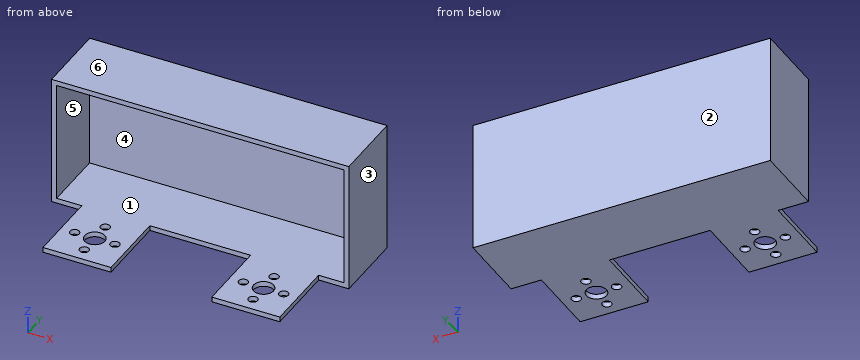
Autodesk Inventor part; units mm, degrees
ref_plane "YZ Plane" through (0, 0, 0) normal (1, 0, 0) x (0, 1, 0)
ref_plane "XZ Plane" through (0, 0, 0) normal (0, 1, 0) x (-1, 0, 0)
ref_plane "XY Plane" through (0, 0, 0) normal (0, 0, 1) x (1, 0, 0)
ref_plane "Work Plane7" through (-37.2167, 31.2213, -6.3329) normal (0, 1, 0) x (1, 0, 0)
sketch "Sketch1" plane through (-37.2167, 31.2213, -6.3329) normal (0, 1, 0) x (1, 0, 0)
  arc A0 (-58.7242, 8.25) -> (-74.6429, -6.8045) centre (-66, 0) ccw
  line L0 (-77, 0) -> (-77, -32.6485)
  arc A1 (-74.6429, -15.1955) -> (-58.7242, -30.25) centre (-66, -22) ccw
  line L1 (-66, -33) -> (-77, -33)
  line L2 (-77, -32.6485) -> (-77, -33)
  line L3 (-77, 0) -> (-77, 11)
  arc A2 (30, -7.5498) -> (14.7242, 8.25) centre (22, 0) ccw
  line L4 (22, 11) -> (-77, 11)
  line L5 (-66, -33) -> (33, -33)
  arc A3 (14.7242, -30.25) -> (30, -14.4502) centre (22, -22) ccw
  line L6 (33, -22) -> (33, -33)
  line L7 (33, -22) -> (33, 11)
  line L8 (22, 11) -> (33, 11)
  line L9 (-79, -32.6485) -> (-79, 0)
  line L10 (-79, 0) -> (-79, 13)
  line L11 (-79, 13) -> (22, 13)
  line L12 (22, 13) -> (35, 13)
  line L13 (35, 13) -> (35, -22)
  line L14 (35, -22) -> (35, -35)
  line L15 (35, -35) -> (-66, -35)
  line L16 (-66, -35) -> (-79, -35)
  line L17 (-79, -35) -> (-79, -32.6485)
  line L18 (-81, 15) -> (-81, 0)
  line L19 (-81, 0) -> (-81, -32.6485)
  line L20 (-81, -32.6485) -> (-81, -37)
  line L21 (-81, -37) -> (-66, -37)
  line L22 (-66, -37) -> (37, -37)
  line L23 (37, -37) -> (37, -22)
  line L24 (37, -22) -> (37, 15)
  line L25 (37, 15) -> (22, 15)
  line L26 (22, 15) -> (-81, 15)
  point P0 (37.2167, -6.3329)
  dimension "d0" = 2
  dimension "d1" = 4
extrude "Extrusion1" add sketch "Sketch1" against normal blind 25 contours L26 L25 L24 L23 L22 L21 L20 L19 L18
extrude "Extrusion2" add sketch "Sketch1" along normal blind 4 contours L4 A2 L7 A3 L5 A1 L0 A0 | A0 L3 L4 | L8 L7 A2 | A1 L1 L2 L0 | L6 L5 A3 | L9 L10 L11 L12 L13 L14 L15 L16 L17 | L26 L25 L24 L23 L22 L21 L20 L19 L18
sketch "Sketch3" plane through (-118.2167, 6.2213, 30.6671) normal (0, 0, 1) x (1, 0, 0)
  point P0 (118.2167, -6.2213)
sketch "Sketch4" plane through (-118.2167, 6.2213, 30.6671) normal (0, 0, 1) x (1, 0, 0)
  point P0 (118.2167, -6.2213)
ref_plane "Work Plane2" through (-37.2167, 6.2213, -6.3329) normal (0, -1, 0) x (1, 0, 0)
sketch "Sketch5" plane through (-37.2167, 6.2213, -6.3329) normal (0, -1, 0) x (1, 0, 0)
  line L0 (35, -13) -> (-79, -13)
  line L1 (35, -13) -> (35, -15)
  line L2 (-81, -15) -> (37, -15)
  line L3 (-79, 35) -> (-79, -13)
  line L4 (-79, -13) -> (-79, -15)
  line L5 (-79, -15) -> (35, -15)
  line L6 (35, -15) -> (25, -15)
  line L7 (25, -15) -> (25, -13)
  line L8 (25, -13) -> (-2, -13)
  line L9 (-2, -13) -> (-2, -15)
  line L10 (25, -15) -> (-2, -15)
  line L11 (-79, -15) -> (-69, -15)
  line L12 (-69, -15) -> (-69, -13)
  line L13 (-69, -13) -> (-42, -13)
  line L14 (-42, -13) -> (-42, -15)
  line L15 (-69, -15) -> (-42, -15)
  point P0 (37.2167, 6.3329)
  point P1 (-2, -15)
  point P2 (25, -15)
  point P3 (-42, -15)
  point P4 (-69, -15)
  dimension "d30" = 10
  dimension "d31" = 27
  dimension "d32" = 10
  dimension "d33" = 27
extrude "Extrusion3" add sketch "Sketch5" along normal blind 29.5 contours L7 L2 L9 L0 | L14 L2 L12 L0
ref_plane "Work Plane3" through (-0.2167, 35.2213, -21.3329) normal (0, 0, -1) x (-1, 0, 0)
sketch "Sketch6" plane through (-0.2167, 35.2213, -21.3329) normal (0, 0, -1) x (-1, 0, 0)
  line L0 (106, -58.5) -> (79, -58.5)
  line L1 (106, -58.5) -> (92.5, -58.5)
  line L2 (92.5, -58.5) -> (92.5, -53)
  circle A0 centre (92.5, -53) radius 1.85
  line L3 (92.5, -53) -> (92.5, -45)
  circle A1 centre (92.5, -45) radius 4
  line L4 (92.5, -45) -> (92.5, -37)
  circle A2 centre (92.5, -37) radius 1.85
  line L5 (92.5, -45) -> (84.5, -45)
  line L6 (93.7399, -45) -> (90.2601, -45)
  line L7 (84.5, -45) -> (100.5, -45)
  circle A3 centre (100.5, -45) radius 1.85
  circle A4 centre (84.5, -45) radius 1.85
  line L8 (79, -29) -> (39, -29)
  line L9 (79, -29) -> (59, -29)
  line L10 (59, -29) -> (59, -58.5)
  circle A5 centre (25.5, -53) radius 1.85
  circle A6 centre (25.5, -45) radius 4
  circle A7 centre (25.5, -37) radius 1.85
  circle A8 centre (17.5, -45) radius 1.85
  circle A9 centre (33.5, -45) radius 1.85
  point P0 (-0.2167, -35.2213)
  dimension "d36" = 5.5
  dimension "d37" = 3.7
  dimension "d38" = 8
  dimension "d39" = 8
  dimension "d40" = 8
  dimension "d41" = 3.7
  dimension "d42" = 8
  dimension "d43" = 16
  dimension "d44" = 3.7
  dimension "d45" = 3.7
  dimension "d46" = 20
extrude "Extrusion4" cut sketch "Sketch6" against normal blind 2.25
properties part number "39057 TETRIX 12V 3000mAH Battery Pack Assembly"
Read the model definition and answer for the solid it produces. Units are mm, in the model's axes. Face numbers are marked on the shaded views. A direction names the side the tool comes from. Coordinates: 2 decimals unless noted, no trailing zeros. Order: outer loops, then holes, each group sorted by start corner. A loop starts at its lowest first (then second) coordinate and runs counter-clockwise, first axis right, second up. Notation, with made-up numbers: (43.25, 82) - (61.25, 82) arc R16 ccw to (61.25, 95) - close; hole circle Ø2 at (65.5, 33). An arc over 180 degrees is marked (long way). Answer as a JSON object with one key per item and string values. Group by question number.
Item 1: Section C-C (x = -108) is taken. Give the vertices of the cut face in (y, z), plus the area to 3 significant figures.
Item 2: Flat-ended cylindrical pins translate along their axes: P1, Ø13, axis at x = -25.72, y = -9.78, coming from the -Z side; P2, Ø1.5, axis at x = -85, z = -16, coming from the -Y side; P3, Ø2, axis at x = -55, z = -20.5, coming from the -Y side; P4, Ø1, axis at y = -13, z = -20, coming from the -X side. Find the tip coordinate at first contact, or state that the pin passes through.
Item 3: Section A-A (y = 30) is taken. Give the vertices of the cut face in (x, z), plus the area to 3 significant figures.
Item 4: A tool of negligible diameter and unlimited length cuts with its end or side. For the marked faces 1 and 2, from which of +Z, -Z, +X, -X, +Y, -Y can it reach the whole face along a straight path? Write none if from no direction.
Item 5: Consider probe 1 along Z at (x, y) = (-82, 21); probe 2 along X at (y, z) = (22, 9.5); probe 3 along Y at (x, z) = (-59, 16.5). Determine where each line is inside the solid, lowest interval first. Write a range as from..to.
Item 6: Section D-D (z = 19) is taken. Give the vertices of the cut face in (x, y).
Item 7: The mould has two halves that part along X. Classify the marked faces 3, 4, 5 and 6: +X half, -X half, draft (parallel to the pull), parting line (faces both ways), or undercut.
Item 8: Section B-B (y = 1.5) is taken. Give the vertices of the cut face in (x, z).
Results are:
{
 "1": {"outline": "(6.22, -21.33) - (35.22, -21.33) - (35.22, 30.67) - (6.22, 30.67) - (6.22, 28.67) - (31.22, 28.67) - (31.22, -19.33) - (6.22, -19.33) - close", "area": "308 mm^2"},
 "2": {"P1": "stops at z = -21.33", "P2": "stops at y = 31.22", "P3": "stops at y = 6.22", "P4": "stops at x = -106.22"},
 "3": {"outline": "(-118.22, -21.33) - (-0.22, -21.33) - (-0.22, 30.67) - (-118.22, 30.67) - close; hole (-116.22, -19.33) - (-2.22, -19.33) - (-2.22, 28.67) - (-116.22, 28.67) - close", "area": "664 mm^2"},
 "4": {"face 1": "-Y", "face 2": "+Z, -Z, +X, -X, +Y"},
 "5": {"probe 1": "z = -21.33..-19.33, 28.67..30.67", "probe 2": "x = -118.22..-116.22, -2.22..-0.22", "probe 3": "y = 31.22..35.22"},
 "6": {"outline": "(-118.22, 6.22) - (-116.22, 6.22) - (-116.22, 31.22) - (-2.22, 31.22) - (-2.22, 6.22) - (-0.22, 6.22) - (-0.22, 35.22) - (-118.22, 35.22) - close"},
 "7": {"face 3": "+X half", "face 4": "undercut", "face 5": "undercut", "face 6": "draft"},
 "8": {"outline": "(-106.22, -21.33) - (-79.22, -21.33) - (-79.22, -19.33) - (-106.22, -19.33) - close; (-39.22, -21.33) - (-12.22, -21.33) - (-12.22, -19.33) - (-39.22, -19.33) - close"}
}
